```python
from build123d import *

# Parameters (mm, degrees)
SKETCH1_W           = 152.4
SKETCH1_H           = 30.48
BOSS_EXTRUDE1_DEPTH = 15.24
SKETCH2_W           = 19.05
SKETCH2_H           = 19.05
BOSS_EXTRUDE2_DEPTH = 152.4
SKETCH3_R           = 2.54
CUT_EXTRUDE1_DEPTH  = 214.273047758
FILLET1_R           = 9.525
FILLET2_R           = 9.525
FILLET3_R           = 9.525
FILLET4_R           = 9.525
FILLET5_R           = 5.08
FILLET6_R           = 5.08
FILLET7_R           = 5.08
FILLET8_R           = 5.08


with BuildPart() as part:
    # Sketch1 → Boss-Extrude1 (new body)
    with BuildSketch(Plane(origin=(0, 0, 0), x_dir=(1, 0, 0), z_dir=(0, 1, 0))):
        with Locations((76.2, 15.24)):
            Rectangle(SKETCH1_W, SKETCH1_H)
    extrude(amount=BOSS_EXTRUDE1_DEPTH)

    # Sketch2 → Boss-Extrude2 (add)
    with BuildSketch(Plane.XZ):
        with Locations((136.525, -15.24)):
            Rectangle(SKETCH2_W, SKETCH2_H)
        with Locations((15.875, -15.24)):
            Rectangle(SKETCH2_W, SKETCH2_H)
    extrude(amount=BOSS_EXTRUDE2_DEPTH)

    # Sketch3 → Cut-Extrude1 (cut, through all)
    with BuildSketch(Plane.ZY.offset(-6.35)):
        with Locations((-15.24, -142.875)):
            Circle(SKETCH3_R)
    extrude(amount=-CUT_EXTRUDE1_DEPTH, mode=Mode.SUBTRACT)

    # Fillet1
    fillet1_edges = [part.edges().sort_by_distance(p)[0] for p in [
        (15.875, -152.4, -5.715),
    ]]
    fillet(fillet1_edges, radius=FILLET1_R)

    # Fillet2
    fillet2_edges = [part.edges().sort_by_distance(p)[0] for p in [
        (15.875, -152.4, -24.765),
    ]]
    fillet(fillet2_edges, radius=FILLET2_R - 0.0001)  # a hair under: the kernel refuses the full size

    # Fillet3
    fillet3_edges = [part.edges().sort_by_distance(p)[0] for p in [
        (136.525, -152.4, -24.765),
    ]]
    fillet(fillet3_edges, radius=FILLET3_R)

    # Fillet4
    fillet4_edges = [part.edges().sort_by_distance(p)[0] for p in [
        (136.525, -152.4, -5.715),
    ]]
    fillet(fillet4_edges, radius=FILLET4_R - 0.0001)  # a hair under: the kernel refuses the full size

    # Fillet5
    fillet5_edges = [part.edges().sort_by_distance(p)[0] for p in [
        (76.2, 15.24, 0),
    ]]
    fillet(fillet5_edges, radius=FILLET5_R)

    # Fillet6
    fillet6_edges = [part.edges().sort_by_distance(p)[0] for p in [
        (76.2, 0, 0),
    ]]
    fillet(fillet6_edges, radius=FILLET6_R)

    # Fillet7
    fillet7_edges = [part.edges().sort_by_distance(p)[0] for p in [
        (76.2, 0, -30.48),
    ]]
    fillet(fillet7_edges, radius=FILLET7_R)

    # Fillet8
    fillet8_edges = [part.edges().sort_by_distance(p)[0] for p in [
        (76.2, 15.24, -30.48),
    ]]
    fillet(fillet8_edges, radius=FILLET8_R)


solid = part.part
```
For this review, take the finished solid that the model builds, in its own axes (mm). A direction names the side the tool comes from. Coordinates: 2 decimals unless noted, no trailing zeros. Order: outer loops, then holes, each group sorted by start corner. A loop starts at its lowest first (then second) coordinate and runs counter-clockwise, first axis right, second up. Notation, with made-up numbers: (86.5, 71) -> (144.5, 71) arc R30 cw to (144.5, 103) -> close; hole circle Ø2 at (26.5, 34.25). An arc over 180 degrees is marked (long way). Use CSV: the item, a comma, the result in double quotes. Start each with the question number.
Item 1: We need section D-D, the plane z = -8.5. Give the boundary of the cut face in (x, y).
Item 2: Draft analysis for pull direction X (two halves, no side actions). For faces 1 (the face through (127, -75, -15)), 2 (the face through (152.4, 8, -15)), 3 (the face through (136, -70, -24.765)), state which applies: pulls with the +X half, pulls with the -X half, needs draft (parallel to the pull), parting line crosses it, or undercut.
Item 3: Insertion check: pin 1 (3 mm diameter, centred on y = -142.875, z = -15.24, fed in from +X); pin 2 (15 mm diameter, centred on y = -95, z = -11, fed in from +X); pin 3 (6 mm diameter, centred on x = 131, y = -125, fed in from -Z) (3 decimals); pin 4 (5.5 mm diameter, centred on x = 133.5, y = -67, fed in from +Z) (3 decimals). Each pin has a flat end and moves straight along its axis. Give the tip position at first contact, or say it passes through.
Item 4: We need section C-C, the plane x = 93. Give the boundary of the cut face in (y, z).
Item 5: Wall thickness on probe 1 along Y at (x, z) = (138, -15.24) (3 decimals); probe 2 along X at (y, z) = (-41, -10.5); probe 3 along Z at (x, y) = (11, -142.5) (3 decimals): over which ranges is each line inside the solid? List them lowest first.
Item 6: For faces 4 (the face through (77.267, 1.449, -28.952)), 5 (the face through (6.35, -75, -15)), 6 (the face through (16, -70, -5.715)), list the 3-axis set-ups (+Z, -Z, +X, -X, +Y, -Y) from which the entire face can be reached by the end or side of a thin tool; tool diameter is ignored.
Item 7: We need section A-A, the plane y = -21.5. Give the boundary of the cut face in (x, z) (3 decimals), then the cut area to 3 significant figures.
Derived:
1,outline,"(0, 0) -> (6.35, 0) -> (6.35, -149.61) -> (25.4, -149.61) -> (25.4, 0) -> (127, 0) -> (127, -149.61) -> (146.05, -149.61) -> (146.05, 0) -> (152.4, 0) -> (152.4, 15.24) -> (0, 15.24) -> close"
2,face 1,"undercut"
2,face 2,"pulls with the +X half"
2,face 3,"needs draft"
3,pin 1,"passes through"
3,pin 2,"stops at x = 146.05"
3,pin 3,"stops at z = -24.765"
3,pin 4,"stops at z = -5.715"
4,outline,"(0, -25.4) arc R5.08 ccw to (5.08, -30.48) -> (10.16, -30.48) arc R5.08 ccw to (15.24, -25.4) -> (15.24, -5.08) arc R5.08 ccw to (10.16, 0) -> (5.08, 0) arc R5.08 ccw to (0, -5.08) -> close"
5,probe 1,"y = -152.4 to -145.415, -140.335 to 15.24"
5,probe 2,"x = 6.35 to 25.4, 127 to 146.05"
5,probe 3,"z = -24.765 to -17.752, -12.728 to -5.715"
6,face 4,"-Z, +X, -X, -Y"
6,face 5,"+Z, -Z, -X, -Y"
6,face 6,"+Z, +X, -X, -Y"
7,outline,"(6.35, -24.765) -> (25.4, -24.765) -> (25.4, -5.715) -> (6.35, -5.715) -> close; (127, -24.765) -> (146.05, -24.765) -> (146.05, -5.715) -> (127, -5.715) -> close"
7,area,"726 mm^2"
